For this review, use the dimensioned drawing (mm, ordinates from the lowest corner) and the shaded views. A direction names the side the tool comes from. Coordinates: 2 decimals unless noted, no trailing zeros. Loops run counter-clockwise (first coordinate to the right, second up) from the corner with the lowest first, then second, coordinate; pieces in that order, holes last. Notation, with made-up numbers: M 38,82.5 L 84,82.5 A10 ccw 84,86.5 Z; hole C 12.5,19.5 d3. An arc over 180 degrees is marked long. One line per item, written item: value.
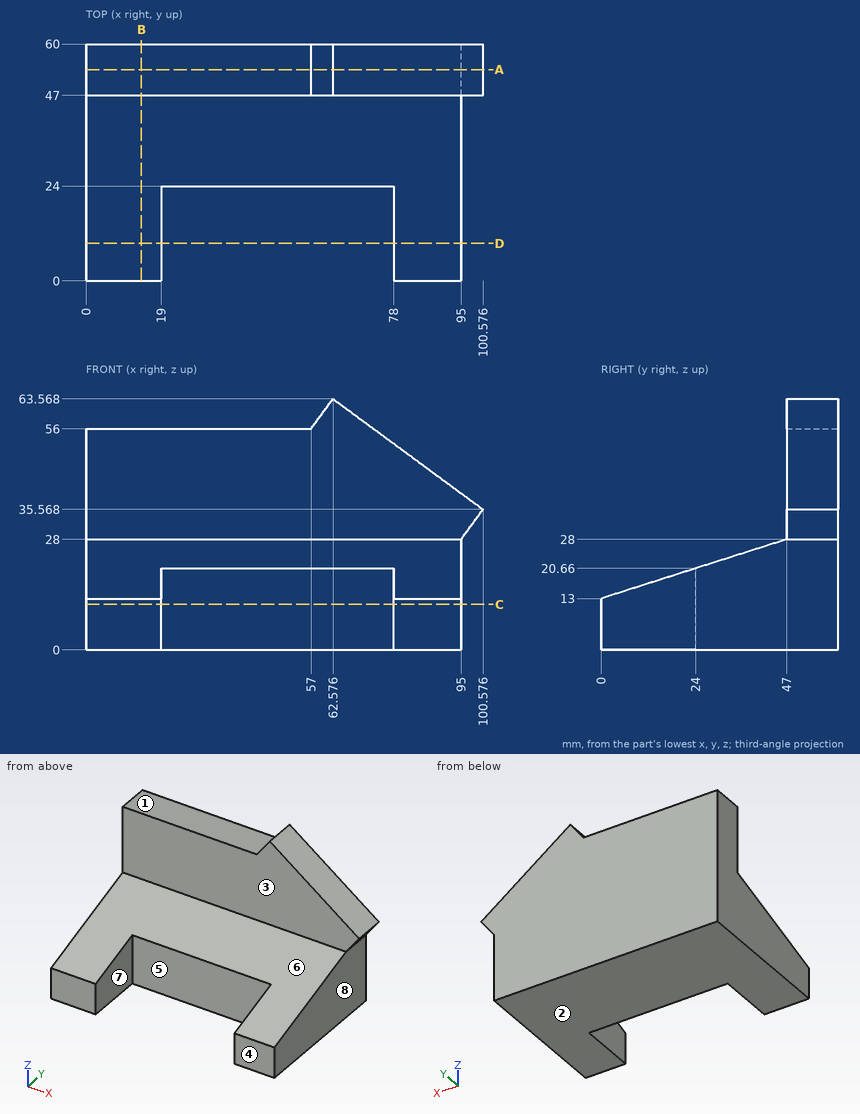
(1) Mouldability with a two-part tool opening along X and no side actions: class the marked faces 6, 7 and 8 as released by +X, released by -X, zero draft, split by the parting line, or undercut.
Reply:
face 6: zero draft
face 7: undercut
face 8: released by +X
(2) To check wall thickness, follow line 1 along Y through (x, z) = (51.5, 48); line 2 along X through (y, z) = (4, 9); line 3 along Z through (x, y) = (38, 55.5). State the ranges of each line that lie inside material, in increasing order. Write a range as [from, to].
Reply:
line 1: y = [47, 60]
line 2: x = [0, 19], [78, 95]
line 3: z = [0, 56]
(3) We need section C-C on z = 11.5. State the section outline as (x, y) points.
Reply:
outline: M 0,0 L 19,0 L 19,24 L 78,24 L 78,0 L 95,0 L 95,60 L 0,60 Z
(4) Tool access review of the marked faces 1, 2, 3, 4 and 5: name each direction out of +Z, -Z, +X, -X, +Y, -Y from which nothing blocks a thin tool from reaching the whole face with its end or side.
Reply:
face 1: +Z, -X, +Y, -Y
face 2: -Z, +X, -X, +Y, -Y
face 3: +Z, +X, -X, -Y
face 4: +Z, -Z, +X, -X, -Y
face 5: +Z, -Z, -Y
(5) Insertion check: pin 1 (16.5 mm diameter, centred on x = 60, z = 5.5, fed in from -Y); pin 2 (4 mm diameter, centred on y = 44, z = 13.5, fed in from +X); pin 3 (10.5 mm diameter, centred on x = 28, y = 51.5, fed in from +Z). Each pin has a flat end and moves straight along its axis. Give the tip position at first contact, or say it passes through.
Reply:
pin 1: stops at y = 24
pin 2: stops at x = 95
pin 3: stops at z = 56
(6) We need section A-A on y = 53.5. State the section outline as (x, z) points.
Reply:
outline: M 0,0 L 95,0 L 95,28 L 100.58,35.57 L 62.58,63.57 L 57,56 L 0,56 Z
(7) We need section D-D on y = 9.5. State the section outline as (x, z) points, then the cut area to 3 significant figures.
Reply:
outline: M 0,0 L 19,0 L 19,16.03 L 0,16.03 Z; M 78,0 L 95,0 L 95,16.03 L 78,16.03 Z
area: 577 mm2
(8) We need section B-B on x = 14. State the section outline as (y, z) points.
Reply:
outline: M 0,0 L 60,0 L 60,56 L 47,56 L 47,28 L 0,13 Z
